Autodesk Inventor part; units mm, degrees
ref_plane "YZ Plane" through (0, 0, 0) normal (1, 0, 0) x (0, 1, 0)
ref_plane "XZ Plane" through (0, 0, 0) normal (0, 1, 0) x (-1, 0, 0)
ref_plane "XY Plane" through (0, 0, 0) normal (0, 0, 1) x (1, 0, 0)
sketch "Skizze1" plane through (0, 0, 0) normal (0, 0, 1) x (1, 0, 0)
  line L0 (-250, 120) -> (250, 120)
  line L1 (250, 120) -> (250, -120)
  line L2 (250, -120) -> (-250, -120)
  line L3 (-250, -120) -> (-250, 120)
  line L4 (-250, 120) -> (250, -120) construction
  line L5 (250, 120) -> (-250, -120) construction
  point P0 (0, 0)
  dimension "d0" = 500
  dimension "d1" = 240
extrude "Extrusion1" add sketch "Skizze1" along normal blind 10
sketch "Skizze3" plane through (0, 0, 0) normal (0, 0, -1) x (-1, 0, 0)
  line L0 (-250, 120) -> (-250, -120)
  line L1 (-250, -120) -> (250, -120)
  line L2 (-156.245, -89) -> (-143.755, -89)
  line L3 (-131, -76.245) -> (-131, -63.755)
  line L4 (-143.755, -51) -> (-156.245, -51)
  line L5 (-169, -63.755) -> (-169, -76.245)
  line L6 (-156.245, -89) -> (-143.755, -51) construction
  line L7 (-131, -76.245) -> (-169, -63.755) construction
  arc A0 (-143.755, -89) -> (-131, -76.245) centre (-150, -70) ccw
  arc A1 (-169, -76.245) -> (-156.245, -89) centre (-150, -70) ccw
  arc A2 (-131, -63.755) -> (-143.755, -51) centre (-150, -70) ccw
  arc A3 (-156.245, -51) -> (-169, -63.755) centre (-150, -70) ccw
  point P0 (0, 0)
  dimension "d32" = 38
  dimension "d33" = 20
  dimension "d34" = 50
  dimension "d35" = 100
extrude "Extrusion3" cut sketch "Skizze3" against normal through all
sketch "Skizze4" plane through (0, 0, 0) normal (0, 0, -1) x (-1, 0, 0)
  arc A0 (-143.755, -89) -> (-131, -76.245) centre (-150, -70) ccw
  line L0 (-134, -86) -> (-166, -86)
  line L1 (-166, -86) -> (-166, -54)
  line L2 (-166, -54) -> (-134, -54)
  line L3 (-134, -54) -> (-134, -86)
  line L4 (-134, -86) -> (-166, -54) construction
  line L5 (-166, -86) -> (-134, -54) construction
  point P0 (0, 0)
  dimension "d38" = 32
  dimension "d39" = 32
hole "Bohrung3" at (134, -54, 0) at (134, -86, 0) at (166, -86, 0) at (166, -54, 0) direction (0, 0, 1) diameter 2.459 end through all
properties part number "Lid_TopPanel" material "Polycarbonat, klar"
Geometry: final body of the model. Coordinates: model frame, mm. A direction names the side the tool comes from. Round coordinates to 2 decimals unless told otherwise and drop trailing zeros. Use one line per item in the form item = value.
Item 1: Draft query along Y for faces 3 (the flat face through (-3, 120, 5)), 4 (the flat face through (-250, -2, 5)), 5 (the flat face through (169, -70, 5)). Return one class per face: released by +Y, released by -Y, zero draft, split by the parting line, or undercut.
Evaluation:
face_3 = released by +Y
face_4 = zero draft
face_5 = undercut
Item 2: Contact query for flat-ended pins moving along their axis: pin 1 Ø2 at (x, y) = (134, -86) entering from +Z; pin 2 Ø3 at (x, y) = (166, -86) entering from -Z. Output: stop coordinate, or through.
Evaluation:
pin_1 = through
pin_2 = 0
Item 3: Access query for faces 1 (the flat face through (-3, 2, 0)), 2 (the cylindrical face through (164.049, -55.766, 4.93)). Directions: +Z, -Z, +X, -X, +Y, -Y. A direction counts if a zero-diameter tool reaches every point of the face in a straight line with its end or side. Return the directions, or none.
Evaluation:
face_1 = -Z, +X, -X, +Y, -Y
face_2 = +Z, -Z
Item 4: Material intervals for probe 1 along X at (y, z) = (-70, 9); probe 2 along X at (y, z) = (-86, 4.5); probe 3 along Y at (x, z) = (140, 3.25), sorted ascending.
Evaluation:
probe_1 = -250 to 131, 169 to 250
probe_2 = -250 to 132.77, 135.23 to 138, 162 to 164.77, 167.23 to 250
probe_3 = -120 to -87.32, -52.68 to 120
